For this review, take the finished solid that the model builds, in its own axes (mm). Round coordinates to 2 decimals unless told otherwise and drop trailing zeros. Loops run counter-clockwise (first coordinate to the right, second up) from the corner with the lowest first, then second, coordinate; pieces in that order, holes last. Notation, with made-up numbers: (63, -9) -> (80, -9) arc R33 ccw to (80, 28) -> close; hole circle Ø3 at (68.25, 28.25). An arc over 180 degrees is marked (long way). Write each question's results on one line, items separated by ' | '.
```python
from build123d import *

# Parameters (mm, degrees)
BOSS_EXTRUDE2_DEPTH = 6
SKETCH3_R           = 3.3
CUT_EXTRUDE1_DEPTH  = 159.587712323
FILLET1_R           = 5


with BuildPart() as part:
    # Sketch1 → Boss-Extrude2 (new body)
    with BuildSketch(Plane(origin=(0, 0, 0), x_dir=(1, 0, 0), z_dir=(0, 1, 0))):
        Polygon((-85, 93.75), (-65, 93.75), (-65, -93.75), (65, -93.75), (65, 93.75), (85, 93.75), (85, 133.75), (-85, 133.75), align=None)
    extrude(amount=BOSS_EXTRUDE2_DEPTH)

    # Sketch3 → Cut-Extrude1 (cut, through all)
    with BuildSketch(Plane(origin=(0, 6, 0), x_dir=(1, 0, 0), z_dir=(0, 1, 0))):
        with Locations(Location((-75, 113.75, 0), (0, 0, 270))):
            Circle(SKETCH3_R)
        with Locations(Location((-32.5, -83.75, 0), (0, 0, 270))):
            Circle(SKETCH3_R)
        with Locations(Location((75, 113.75, 0), (0, 0, 90))):
            Circle(SKETCH3_R)
        with Locations(Location((32.5, -83.75, 0), (0, 0, 90))):
            Circle(SKETCH3_R)
    extrude(amount=-CUT_EXTRUDE1_DEPTH, mode=Mode.SUBTRACT)

    # Fillet1
    fillet1_edges = [part.edges().sort_by_distance(p)[0] for p in [
        (65, 3, -93.75),
        (65, 3, 93.75),
        (-65, 3, 93.75),
        (-65, 3, -93.75),
        (-85, 3, -93.75),
        (-85, 3, -133.75),
        (85, 3, -133.75),
        (85, 3, -93.75),
    ]]
    fillet(fillet1_edges, radius=FILLET1_R)


solid = part.part
```
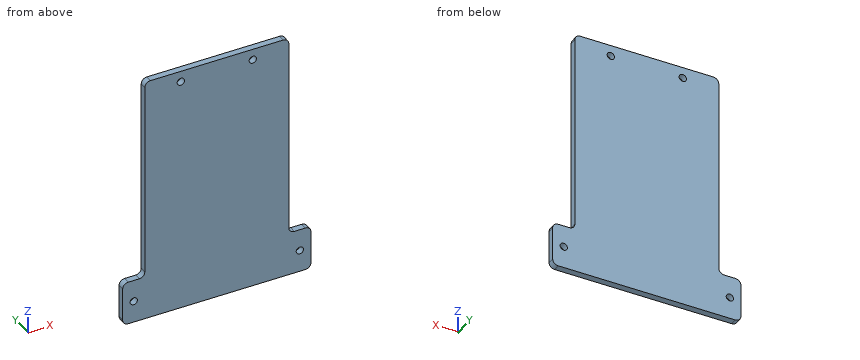
1. For pin 1 (1.8 mm diameter, centred on y = 2, z = -34, fed in from +X); pin 2 (1.8 mm diameter, centred on x = -73, y = 1.5, fed in from +Z), all flat-tipped, find the tip position at first contact; note any pin that passes through.
Values found:
pin 1: stops at x = 65 | pin 2: stops at z = -93.75
2. To check wall thickness, follow probe 1 along X at (y, z) = (2.2, -113.75); probe 2 along X at (y, z) = (1.3, 83.75); probe 3 along Z at (x, y) = (32.5, 1.55). State the ranges of each line that lie inside material, in increasing order.
Values found:
probe 1: x = -85 to -78.3, -71.7 to 71.7, 78.3 to 85 | probe 2: x = -65 to -35.8, -29.2 to 29.2, 35.8 to 65 | probe 3: z = -133.75 to 80.45, 87.05 to 93.75
3. Consider section B-B (x = 32.5). State the section outline as (y, z) points, plus the area to 3 significant figures.
Values found:
outline: (0, -133.75) -> (6, -133.75) -> (6, 80.45) -> (0, 80.45) -> close; (0, 87.05) -> (6, 87.05) -> (6, 93.75) -> (0, 93.75) -> close | area: 1,330 mm2
4. Consider section A-A (z = 83.75). State the section outline as (x, y) points.
Values found:
outline: (-65, 0) -> (-35.8, 0) -> (-35.8, 6) -> (-65, 6) -> close; (-29.2, 0) -> (29.2, 0) -> (29.2, 6) -> (-29.2, 6) -> close; (35.8, 0) -> (65, 0) -> (65, 6) -> (35.8, 6) -> close
5. Consider section D-D (z = -113.75). State the section outline as (x, y) points, plus the area to 3 significant figures.
Values found:
outline: (-85, 0) -> (-78.3, 0) -> (-78.3, 6) -> (-85, 6) -> close; (-71.7, 0) -> (71.7, 0) -> (71.7, 6) -> (-71.7, 6) -> close; (78.3, 0) -> (85, 0) -> (85, 6) -> (78.3, 6) -> close | area: 941 mm2
6. Consider section C-C (y = 3.1). State the section outline as (x, z) points.
Values found:
outline: (-85, -128.75) arc R5 ccw to (-80, -133.75) -> (80, -133.75) arc R5 ccw to (85, -128.75) -> (85, -98.75) arc R5 ccw to (80, -93.75) -> (70, -93.75) arc R5 cw to (65, -88.75) -> (65, 88.75) arc R5 ccw to (60, 93.75) -> (-60, 93.75) arc R5 ccw to (-65, 88.75) -> (-65, -88.75) arc R5 cw to (-70, -93.75) -> (-80, -93.75) arc R5 ccw to (-85, -98.75) -> close; hole circle Ø6.6 at (-75, -113.75); hole circle Ø6.6 at (-32.5, 83.75); hole circle Ø6.6 at (32.5, 83.75); hole circle Ø6.6 at (75, -113.75)
